Check sheet for the modelled part. Datum: model origin and axes. Units: mm. Face numbers are marked on the shaded views. A direction names the side the tool comes from. Coordinates: 2 decimals unless noted, no trailing zeros. Order: outer loops, then holes, each group sorted by start corner. A loop starts at its lowest first (then second) coordinate and runs counter-clockwise, first axis right, second up. Notation, with made-up numbers: (29.25, -10.75) -> (35.25, -10.75) arc R25 cw to (35.25, 5.25) -> close; hole circle Ø6 at (49, -8.75). An arc over 180 degrees is marked (long way). Put each result on its own line as item: value. Start each with the question number.
```python
from build123d import *

# Parameters (mm, degrees)
SKETCH1_W           = 24
SKETCH1_H           = 16
BOSS_EXTRUDE1_DEPTH = 16
SKETCH2_R           = 5.571856639
BOSS_EXTRUDE2_DEPTH = 3
FILLET1_R           = 1
FILLET2_R           = 1
FILLET3_R           = 1


with BuildPart() as part:
    # Sketch1 → Boss-Extrude1 (new body)
    with BuildSketch(Plane(origin=(0, 0, 0), x_dir=(1, 0, 0), z_dir=(0, 1, 0))):
        Rectangle(SKETCH1_W, SKETCH1_H)
    extrude(amount=BOSS_EXTRUDE1_DEPTH)

    # Sketch2 → Boss-Extrude2 (add)
    with BuildSketch(Plane(origin=(0, 16, 0), x_dir=(1, 0, 0), z_dir=(0, 1, 0))):
        with Locations(Location((0, 0, 0), (0, 0, 270))):
            Circle(SKETCH2_R)
    extrude(amount=BOSS_EXTRUDE2_DEPTH)

    # Sketch4 → Revolve1 (revolve)
    with BuildSketch(Plane.XY):
        Polygon((0, 19), (8, 19), (8, 25), (2.5, 25), (2.5, 37), (0, 37), align=None)
    revolve(axis=Axis((0, 0, 0), (0, 1, 0)))

    # Fillet1
    fillet1_edges = [part.edges().sort_by_distance(p)[0] for p in [
        (-8, 25, 0),
    ]]
    fillet(fillet1_edges, radius=FILLET1_R)

    # Fillet2
    fillet2_edges = [part.edges().sort_by_distance(p)[0] for p in [
        (-2.5, 37, 0),
    ]]
    fillet(fillet2_edges, radius=FILLET2_R)

    # Fillet3
    fillet3_edges = [part.edges().sort_by_distance(p)[0] for p in [
        (12, 8, 8),
        (-12, 8, 8),
        (-12, 8, -8),
        (12, 8, -8),
    ]]
    fillet(fillet3_edges, radius=FILLET3_R)


solid = part.part
```
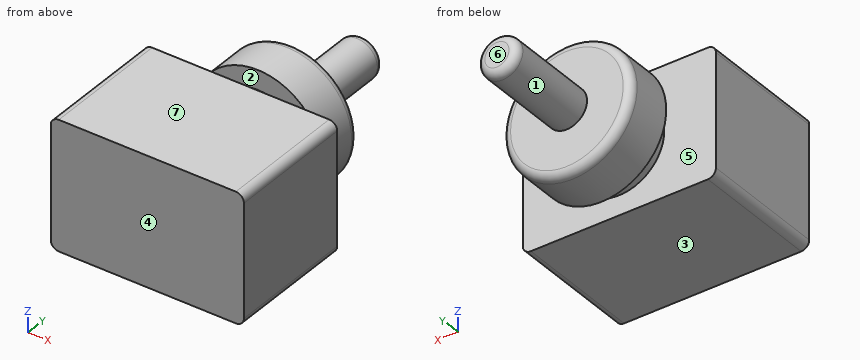
1) Sectioned sample at A-A (x = 0). Record the boundary of the cut face in (y, z).
2) Gauge pin test, flat ends, axial feed: pin 1 (10 mm diameter, centred on x = -6.5, y = 18, fed in from +Z); pin 2 (2 mm diameter, centred on x = 8, y = 27.5, fed in from +Z); pin 3 (8 mm diameter, centred on x = -5.5, z = 2.5, fed in from +Y). Record the tip position at first contact, or that the pin passes through.
3) Sectioned sample at B-B (z = 0). Record the boundary of the cut face in (x, y), plus the area to 3 significant figures.
4) Sectioned sample at C-C (y = 20). Record the boundary of the cut face in (x, z).
5) Scan lines: line 1 along Y through (x, z) = (-5.5, 3.25); line 2 along X through (y, z) = (26, 0); line 3 along Y through (x, z) = (2.75, -4). Record each from-to range of solid material in increasing order. Write a range as [from, to].
6) Mould release check, pull along Y, two halves, no side actions. Record for the marked faces 4, 5, 6 and 7: +Y half, -Y half, draft (parallel to the pull), parting line (faces both ways), or undercut.
7) Access from +Z, -Z, +X, -X, +Y, -Y to the whole of each face (thin tool, end or side, straight path). Record for the marked faces 1, 2 and 3.
8) Sectioned sample at D-D (y = 32.5). Record the boundary of the cut face in (x, z), plus the area to 3 significant figures.
Entries:
1. outline: (0, -8) -> (16, -8) -> (16, -5.57) -> (19, -5.57) -> (19, -8) -> (24, -8) arc R1 ccw to (25, -7) -> (25, -2.5) -> (36, -2.5) arc R1 ccw to (37, -1.5) -> (37, 1.5) arc R1 ccw to (36, 2.5) -> (25, 2.5) -> (25, 7) arc R1 ccw to (24, 8) -> (19, 8) -> (19, 5.57) -> (16, 5.57) -> (16, 8) -> (0, 8) -> close
2. pin 1: stops at z = 8
2. pin 2: passes through
2. pin 3: stops at y = 36.84
3. outline: (-12, 0) -> (12, 0) -> (12, 16) -> (5.57, 16) -> (5.57, 19) -> (8, 19) -> (8, 24) arc R1 ccw to (7, 25) -> (2.5, 25) -> (2.5, 36) arc R1 ccw to (1.5, 37) -> (-1.5, 37) arc R1 ccw to (-2.5, 36) -> (-2.5, 25) -> (-7, 25) arc R1 ccw to (-8, 24) -> (-8, 19) -> (-5.57, 19) -> (-5.57, 16) -> (-12, 16) -> close
3. area: 573 mm2
4. outline: circle Ø16 at (0, 0)
5. line 1: y = [0, 16], [19, 25]
5. line 2: x = [-2.5, 2.5]
5. line 3: y = [0, 25]
6. face 4: -Y half
6. face 5: undercut
6. face 6: +Y half
6. face 7: draft
7. face 1: +Y
7. face 2: none
7. face 3: -Z, +X, -X, +Y, -Y
8. outline: circle Ø5 at (0, 0)
8. area: 19.6 mm2
